Geometry check sheet. Reference: the model listing, model coordinates, mm. Round coordinates to 2 decimals unless told otherwise and drop trailing zeros. Loops run counter-clockwise (first coordinate to the right, second up) from the corner with the lowest first, then second, coordinate; pieces in that order, holes last. Notation, with made-up numbers: (-13.75, -35) - (18.25, -35) arc R16 cw to (18.25, -17) - close; hole circle Ø5 at (61, -11). An arc over 180 degrees is marked (long way). Write item = value, one per line.
Autodesk Inventor part; units mm, degrees
ref_plane "YZ Plane" through (0, 0, 0) normal (1, 0, 0) x (0, 1, 0)
ref_plane "XZ Plane" through (0, 0, 0) normal (0, 1, 0) x (-1, 0, 0)
ref_plane "XY Plane" through (0, 0, 0) normal (0, 0, 1) x (1, 0, 0)
sketch "Sketch1" plane through (0, 0, 0) normal (0, 1, 0) x (-1, 0, 0)
  line L0 (0, 0) -> (-5.3, 0)
  line L1 (-5.3, 0) -> (-5.3, -3.3)
  line L2 (-5.3, -3.3) -> (0, -3.3)
  line L3 (0, -3.3) -> (0, 0)
  line L4 (0, -66.3) -> (-5.3, -66.3)
  line L5 (-5.3, -66.3) -> (-5.3, -69.6)
  line L6 (-5.3, -69.6) -> (0, -69.6)
  line L7 (0, -69.6) -> (0, -66.3)
  dimension "d0" = 5.3
  dimension "d1" = 3.3
  dimension "d2" = 63
  dimension "d3" = 5.3
  dimension "d4" = 3.3
sketch "Sketch1 outline for Rails" plane through (0, 0, 0) normal (0, 1, 0) x (-1, 0, 0)
  line L0 (0, -66.3) -> (-5.3, -66.3)
  line L1 (0, -69.6) -> (0, -66.3)
  line L2 (-5.3, -69.6) -> (0, -69.6)
  line L3 (-5.3, -66.3) -> (-5.3, -69.6)
  line L4 (0, 0) -> (-5.3, 0)
  line L5 (0, -3.3) -> (0, 0)
  line L6 (-5.3, -3.3) -> (0, -3.3)
  line L7 (-5.3, 0) -> (-5.3, -3.3)
extrude "Rails" add sketch "Sketch1 outline for Rails" along normal blind 70
sketch "Sketch2" plane through (0, 70, 0) normal (0, 1, 0) x (1, 0, 0)
  line L0 (0, 0) -> (5.3, 0)
  line L1 (5.3, 66.3) -> (5.3, 69.6)
  line L2 (2.65, 0) -> (5.3, 0)
  line L3 (5.3, 0) -> (5.3, 69.6)
  line L4 (5.3, 69.6) -> (2.65, 69.6)
  line L5 (2.65, 69.6) -> (2.65, 0)
sketch "Sketch2 outline for Extrusion2" plane through (0, 70, 0) normal (0, 1, 0) x (1, 0, 0)
  line L0 (5.3, 69.6) -> (2.65, 69.6)
  line L1 (5.3, 66.3) -> (5.3, 69.6)
  line L2 (5.3, 0) -> (5.3, 66.3)
  line L3 (2.65, 0) -> (5.3, 0)
  line L4 (2.65, 69.6) -> (2.65, 0)
extrude "Extrusion2" add sketch "Sketch2 outline for Extrusion2" along normal blind 5
chamfer "Chamfer1" distance 2.6 angle 45 1 edges at (2.65, 75, -34.8)
fillet "Scoop lip" radius 9 1 edges at (2.65, 72.4, -34.8)
fillet "Purely Aesthetics" radius 12 2 edges at (0, 70, -1.65) (0, 70, -67.95)
sketch "Sketch4" plane through (0, 0, 0) normal (0, 0, 1) x (1, 0, 0)
  circle A0 centre (2.577408, 3.76) radius 1
  circle A1 centre (2.577408, 7.447823) radius 1
  circle A2 centre (2.577408, 11.422475) radius 1
  circle A3 centre (2.577408, 15.602007) radius 1
  circle A4 centre (2.577408, 19.740564) radius 1
  circle A5 centre (2.577408, 23.674241) radius 1
  circle A6 centre (2.577408, 27.68987) radius 1
  circle A7 centre (2.577408, 31.541595) radius 1
  circle A8 centre (2.577408, 35.516248) radius 1
  circle A9 centre (2.577408, 39.736756) radius 1
  circle A10 centre (2.577408, 43.547506) radius 1
  circle A11 centre (2.577408, 47.727037) radius 1
  circle A12 centre (2.577408, 52.234376) radius 1
  circle A13 centre (2.577408, 57.766109) radius 1
  circle A14 centre (2.577408, 62.191496) radius 1
  circle A15 centre (2.577408, 65.715415) radius 1
  point P0 (0, 0)
  dimension "d14" = 2
  dimension "d15" = 2
  dimension "d16" = 2
  dimension "d17" = 2
  dimension "d18" = 2
  dimension "d19" = 2
  dimension "d20" = 2
  dimension "d21" = 2
  dimension "d22" = 2
  dimension "d23" = 2
  dimension "d24" = 2
  dimension "d25" = 2
  dimension "d26" = 2
  dimension "d27" = 2
  dimension "d28" = 2
  dimension "d29" = 2
sketch "Sketch4 outline for Mesh Mounting Holes" plane through (0, 0, 0) normal (0, 0, 1) x (1, 0, 0)
  circle A0 centre (2.577408, 65.715415) radius 1
  circle A1 centre (2.577408, 62.191496) radius 1
  circle A2 centre (2.577408, 57.766109) radius 1
  circle A3 centre (2.577408, 52.234376) radius 1
  circle A4 centre (2.577408, 47.727037) radius 1
  circle A5 centre (2.577408, 43.547506) radius 1
  circle A6 centre (2.577408, 39.736756) radius 1
  circle A7 centre (2.577408, 35.516248) radius 1
  circle A8 centre (2.577408, 31.541595) radius 1
  circle A9 centre (2.577408, 27.68987) radius 1
  circle A10 centre (2.577408, 23.674241) radius 1
  circle A11 centre (2.577408, 19.740564) radius 1
  circle A12 centre (2.577408, 15.602007) radius 1
  circle A13 centre (2.577408, 11.422475) radius 1
  circle A14 centre (2.577408, 7.447823) radius 1
  circle A15 centre (2.577408, 3.76) radius 1
extrude "Mesh Mounting Holes" cut sketch "Sketch4 outline for Mesh Mounting Holes" against normal blind 70
properties part number "rails+scoop"
(1) Gauge pin test, flat end, axial feed: pin 1 (2 mm diameter, centred on x = 3, z = -25, fed in from +Y). Record the tip position at first contact, or that the pin passes through.
Answers follow:
pin_1 = 73.48
(2) Section check B-B (z = -53). Enter the section's corners in (x, y).
Answers follow:
outline = (2.65, 70) - (5.3, 70) - (5.3, 75) - (5.25, 75) - (5.17, 74.92) arc R9 ccw to start
(3) Section check A-A (y = 3.76). Enter the section's corners in (x, z).
Answers follow:
outline = (0, -69.6) - (1.58, -69.6) - (1.58, -66.3) - (0, -66.3) - close; (0, -3.3) - (1.58, -3.3) - (1.58, 0) - (0, 0) - close; (3.58, -69.6) - (5.3, -69.6) - (5.3, -66.3) - (3.58, -66.3) - close; (3.58, -3.3) - (5.3, -3.3) - (5.3, 0) - (3.58, 0) - close
(4) Section check C-C (y = 69). Enter the section's corners in (x, z).
Answers follow:
outline = (1.93, -69.6) - (5.3, -69.6) - (5.3, -66.3) - (1.93, -66.3) - close; (1.93, -3.3) - (5.3, -3.3) - (5.3, 0) - (1.93, 0) - close
(5) Scan lines: L1, parallel to Z at x = 0.6, y = 14; L2, parallel to Y at x = 3.7, z = -43; L3, parallel to Y at x = 3.55, z = -41.5. Record each from-to range of solid material in increasing order. Write a range as [from, to].
Answers follow:
L1 = [-69.6, -66.3], [-3.3, 0]
L2 = [70, 72.99]
L3 = [70, 72.71]
(6) Mould release check, pull along Y, two halves, no side actions. Record for faces 1 (the cylindrical face through (0.663, 66.412, -67.973)), 2 (the cylindrical face through (2.36, 38.76, -1.63)), 3 (the flat face through (3, 37, 0)): pulls with the +Y half, pulls with the -Y half, needs draft (parallel to the pull), parting line crosses it, or undercut.
Answers follow:
face_1 = pulls with the +Y half
face_2 = undercut
face_3 = needs draft
